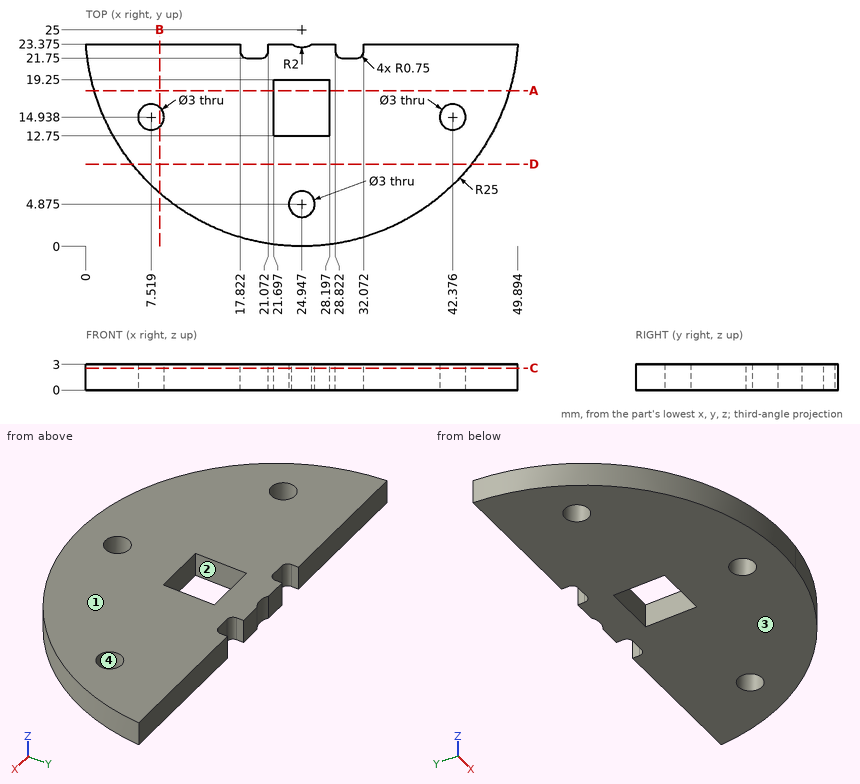
Source: three-view drawing plus pictorial views. Frame: mm from the lowest corner of the part. A direction names the side the tool comes from. Round coordinates to 2 decimals unless told otherwise and drop trailing zeros. Order: outer loops, then holes, each group sorted by start corner. A loop starts at its lowest first (then second) coordinate and runs counter-clockwise, first axis right, second up. Notation, with made-up numbers: (30, 77.5) -> (36, 77.5) arc R11 cw to (36, 98.5) -> close; hole circle Ø10 at (35.5, 47.25). An arc over 180 degrees is marked (long way). Use one line per item in the form item = value.
(1) Section A-A on y = 18. Return loops of the section in (x, z).
Results list:
outline = (0.95, 0) -> (21.7, 0) -> (21.7, 3) -> (0.95, 3) -> close; (28.2, 0) -> (48.95, 0) -> (48.95, 3) -> (28.2, 3) -> close
(2) Section D-D on y = 9.5. Return loops of the section in (x, z), and give its area (3 significant figures).
Results list:
outline = (5.33, 0) -> (44.56, 0) -> (44.56, 3) -> (5.33, 3) -> close
area = 118 mm^2
(3) First-contact query: pin 1 Ø0.7 at (y, z) = (23, 1.5) entering from +X; pin 2 Ø5 at (x, y) = (7.52, 14.94) entering from +Z; pin 3 Ø0.9 at (x, z) = (19.5, 1) entering from +Y. Flat tips, straight axial feed; report the tip coordinate or a pass-through.
Results list:
pin_1 = 49.89
pin_2 = 3
pin_3 = 21.75
(4) Section B-B on x = 8.5. Return loops of the section in (y, z) (1 decimal).
Results list:
outline = (6.2, 0) -> (13.8, 0) -> (13.8, 3) -> (6.2, 3) -> close; (16.1, 0) -> (23.4, 0) -> (23.4, 3) -> (16.1, 3) -> close
(5) Section C-C on z = 2.55. Count the separate pieces of the cut face and the enclosed holes in it.
Results list:
separate_pieces = 1
enclosed_holes = 4
(6) Ray query, probe 1 along X at (y, z) = (3.75, 2.2) (1 decimal); probe 2 along X at (y, z) = (17, 2.3); probe 3 along Y at (x, z) = (15, 0.65) (1 decimal). Return the intervals inside material, ascending. Write a range as [from, to].
Results list:
probe_1 = [11.8, 24], [25.9, 38.1]
probe_2 = [1.26, 21.7], [28.2, 48.63]
probe_3 = [2.1, 23.4]
(7) Draft query along Y for the marked faces 3 and 4. Return one class per face: pulls with the +Y half, pulls with the -Y half, needs draft (parallel to the pull), parting line crosses it, or undercut.
Results list:
face_3 = needs draft
face_4 = undercut
(8) Access query for the marked faces 1 and 2. Directions: +Z, -Z, +X, -X, +Y, -Y. A direction counts if a zero-diameter tool reaches every point of the face in a straight line with its end or side. Return the directions, or none.
Results list:
face_1 = +Z, +X, -X, +Y, -Y
face_2 = +Z, -Z
